Input: part model. Units: mm. Frame: model coordinates. Face numbers are marked on the shaded views. A direction names the side the tool comes from. Coordinates: 2 decimals unless noted, no trailing zeros. Loops run counter-clockwise (first coordinate to the right, second up) from the corner with the lowest first, then second, coordinate; pieces in that order, holes last. Notation, with made-up numbers: (83, 47) - (138, 47) arc R28 cw to (138, 65) - close; hole circle Ø10 at (40.25, 69). An arc over 180 degrees is marked (long way). Use a Markdown table: item, result. Add a question column.
1. Contact query for flat-ended pins moving along their axis: P1, Ø12, axis at x = -24.5, z = 9.5, coming from the +Y side; P2, Ø1.5, axis at y = -6.5, z = -17.5, coming from the -X side; P3, Ø22.5, axis at x = -56, z = -1.5, coming from the -Y side. Output: stop coordinate, or through.
2. Ray query, L1, parallel to X at y = 13.5, z = 17.5; L2, parallel to Y at x = -54, z = -7.5; L3, parallel to Y at x = -43.5, z = -21. Return the intervals inside material, ascending. Write a range as [from, to].
3. Draft query along Z for the marked faces 1, 2 and 3. Return one class per face: released by +Z, released by -Z, zero draft, split by the parting line, or undercut.
4. Access query for the marked faces 4 and 5. Directions: +Z, -Z, +X, -X, +Y, -Y. A direction counts if a zero-diameter tool reaches every point of the face in a straight line with its end or side. Return the directions, or none.
5. Section query D-D on z = 18. Return the cut outline in (x, y), then the cut area to 3 significant figures.
6. Section query B-B on y = -9.5. Return the cut outline in (x, z), then the cut area to 3 significant figures.
7. Section query C-C on x = -29.5. Return the cut outline in (y, z), then the cut area to 3 significant figures.
8. Section query A-A on z = -13. Return the cut outline in (x, y), then the cut area to 3 significant figures.
```python
from build123d import *

# Parameters (mm, degrees)
F2_DEPTH = 15
F3_W     = 24.9072536826
F3_H     = 45.3870967031
F4_DEPTH = 50
F5_DEPTH = 1


# Not quite as in the source:
# - the program builds the solid bodies; features that only make, move or delete a surface that nothing else refers to are left out


with BuildPart() as f2:
    # F0 (on Front) → F2 (new body)
    with BuildSketch(Plane.XZ):
        with BuildLine():
            ThreePointArc((-58.766130358, 22.6935483515), (-42.7193684294, 16.0467619285), (-36.0725820065, 0))
            ThreePointArc((-36.0725820065, 0), (-42.7193684294, -16.0467619285), (-58.766130358, -22.6935483515))
            Line((-58.766130358, -22.6935483515), (36.0725782812, -22.6935483515))
            Line((36.0725782812, -22.6935483515), (36.0725782812, 22.6935483515))
            Line((36.0725782812, 22.6935483515), (-58.766130358, 22.6935483515))
        make_face()
    extrude(amount=F2_DEPTH)

    # F3 (on face) → F4 (join)
    with BuildSketch(Plane.XZ.offset(15)):
        with Locations((23.6189514399, 0)):
            Rectangle(F3_W, F3_H)
    extrude(amount=-F4_DEPTH)

    # F0 (on Front) → F5 (join)
    with BuildSketch(Plane.XZ):
        with BuildLine():
            ThreePointArc((-58.766130358, -22.6935483515), (-42.7193684294, -16.0467619285), (-36.0725820065, 0))
            ThreePointArc((-36.0725820065, 0), (-42.7193684294, 16.0467619285), (-58.766130358, 22.6935483515))
            Line((-58.766130358, 22.6935483515), (-58.766130358, -22.6935483515))
        make_face()
        with BuildLine():
            Line((-58.766130358, -22.6935483515), (-58.766130358, 22.6935483515))
            ThreePointArc((-58.766130358, 22.6935483515), (-81.4596787095, 0), (-58.766130358, -22.6935483515))
        make_face()
    extrude(amount=F5_DEPTH)


solid = f2.part
```
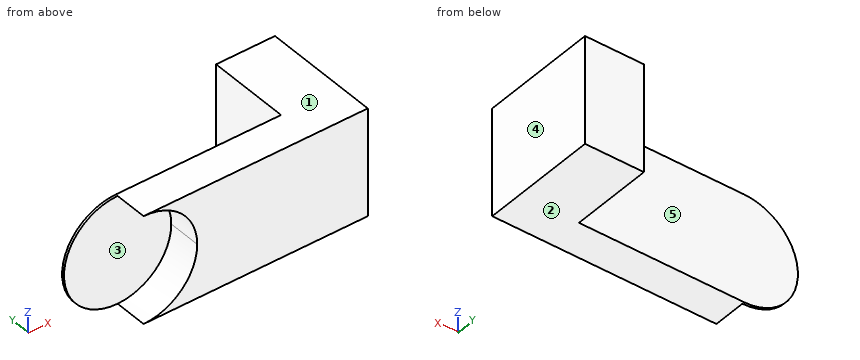
Resolved:
| question | item | result |
|---|---|---|
| 1 | P1 | y = 0 |
| 1 | P2 | x = -45.28 |
| 1 | P3 | y = -1 |
| 2 | L1 | [11.17, 36.07] |
| 2 | L2 | [-1, 0] |
| 2 | L3 | [-15, 0] |
| 3 | face 1 | released by +Z |
| 3 | face 2 | released by -Z |
| 3 | face 3 | undercut |
| 4 | face 4 | +Z, -Z, +X, +Y, -Y |
| 4 | face 5 | +Z, -Z, -X, +Y |
| 5 | outline | (-72.59, -1) - (-44.95, -1) - (-44.95, -15) - (36.07, -15) - (36.07, 35) - (11.17, 35) - (11.17, 0) - (-72.59, 0) - close |
| 5 | area | 2,110 mm² |
| 6 | outline | (-58.77, -22.69) - (36.07, -22.69) - (36.07, 22.69) - (-58.77, 22.69) arc R22.69 cw to start |
| 6 | area | 3,500 mm² |
| 7 | outline | (-15, -22.69) - (0, -22.69) - (0, 22.69) - (-15, 22.69) - close |
| 7 | area | 681 mm² |
| 8 | outline | (-77.37, -1) - (-40.17, -1) - (-40.17, -15) - (36.07, -15) - (36.07, 35) - (11.17, 35) - (11.17, 0) - (-77.37, 0) - close |
| 8 | area | 2,050 mm² |
